```python
from build123d import *

# Parameters (mm, degrees)
SKETCH1_R           = 10
BOSS_EXTRUDE1_DEPTH = 12.5
CUT_EXTRUDE1_DEPTH  = 10
CUT_EXTRUDE2_DEPTH  = 0.5
CHAMFER1_SIZE       = 1


with BuildPart() as part:
    # Sketch1 → Boss-Extrude1 (new body)
    with BuildSketch(Plane(origin=(0, 0, 0), x_dir=(1, 0, 0), z_dir=(0, 1, 0))):
        Circle(SKETCH1_R)
    extrude(amount=BOSS_EXTRUDE1_DEPTH)

    # Sketch2 → Cut-Extrude1 (cut)
    with BuildSketch(Plane.XZ):
        with BuildLine():
            Line((-2.598076211, 1.5), (2.598076211, 1.5))
            ThreePointArc((2.598076211, 1.5), (0, -3), (-2.598076211, 1.5))
        make_face()
    extrude(amount=-CUT_EXTRUDE1_DEPTH, mode=Mode.SUBTRACT)

    # Sketch3 → Cut-Extrude2 (cut)
    with BuildSketch(Plane(origin=(0, 12.5, 0), x_dir=(1, 0, 0), z_dir=(0, 1, 0))):
        Polygon((-1, 7.1), (0, 8.6), (1, 7.1), align=None)
    extrude(amount=-CUT_EXTRUDE2_DEPTH, mode=Mode.SUBTRACT)

    # Chamfer1
    chamfer1_edges = [part.edges().sort_by_distance(p)[0] for p in [
        (-10, 12.5, 0),
    ]]
    chamfer(chamfer1_edges, length=CHAMFER1_SIZE)


solid = part.part
```
Source: CAD feature listing. Evaluate the final solid. Frame: model axes, mm. A direction names the side the tool comes from. Coordinates: 2 decimals unless noted, no trailing zeros. Loops run counter-clockwise (first coordinate to the right, second up) from the corner with the lowest first, then second, coordinate; pieces in that order, holes last. Notation, with made-up numbers: (24, 79.25) - (63, 79.25) arc R27 cw to (63, 101.25) - close; hole circle Ø2 at (17.25, 23). An arc over 180 degrees is marked (long way). Answer as CSV lines item,"result".
1. Reachability of faces 1 (the flat face through (-0.507, 12.254, -7.84)), 2 (the flat face through (0, 5, 1.5)), 3 (the flat face through (0, 12.5, 0)) from +Z, -Z, +X, -X, +Y, -Y: full face, straight path, thin tool, end or side. Return the list, or none.
Established:
face 1,"+Y"
face 2,"-Y"
face 3,"+Z, -Z, +X, -X, +Y"
2. Section A-A (z = 0). Return loops of the section in (x, y).
Established:
outline,"(-10, 0) - (-3, 0) - (-3, 10) - (3, 10) - (3, 0) - (10, 0) - (10, 11.5) - (9, 12.5) - (-9, 12.5) - (-10, 11.5) - close"
3. Section C-C (y = 11). Return loops of the section in (x, z).
Established:
outline,"circle Ø20 at (0, 0)"
4. Contact query for flat-ended pins moving along their axis: pin 1 (3 mm diameter, centred on y = 5.5, z = 6, fed in from -X); pin 2 (1.5 mm diameter, centred on y = 8, z = 7.5, fed in from +X); pin 3 (1.5 mm diameter, centred on y = 7.5, z = -2.5, fed in from -X). Output: stop coordinate, or through.
Established:
pin 1,"stops at x = -8.93"
pin 2,"stops at x = 7.38"
pin 3,"stops at x = -9.85"
5. Ray query, line 1 (Z direction, x = 0, y = 3.5); line 2 (X direction, y = 3.75, z = 0); line 3 (Z direction, x = -1, y = 4.75). Return the intervals inside material, ascending.
Established:
line 1,"z = -10 to -3, 1.5 to 10"
line 2,"x = -10 to -3, 3 to 10"
line 3,"z = -9.95 to -2.83, 1.5 to 9.95"
6. Mould query, pull axis X, two halves, no side actions, for faces 4 (the cylindrical face through (-2.17, 5.67, 9.76)), 5 (the flat face through (0.493, 12.254, -7.86)), 6 (the flat face through (0, 0, 2)). Classes: released by +X, released by -X, zero draft, split by the parting line, or undercut.
Established:
face 4,"split by the parting line"
face 5,"undercut"
face 6,"zero draft"
7. Section B-B (y = 4.5). Return loops of the section in (x, z).
Established:
outline,"circle Ø20 at (0, 0); hole (-2.6, 1.5) arc R3 ccw (long way) to (2.6, 1.5) - close"
